Can you work these out from the drawing? Everything is in mm from the part's minimum corner. A direction names the side the tool comes from. Coordinates: 2 decimals unless noted, no trailing zeros. Order: outer loops, then holes, each group sorted by start corner. A loop starts at its lowest first (then second) coordinate and runs counter-clockwise, first axis right, second up. Notation, with made-up numbers: (31.5, 79.25) - (43.5, 79.25) arc R17 cw to (43.5, 94.25) - close; hole circle Ø1 at (1.25, 4). An arc over 180 degrees is marked (long way). Use CSV: the item, a comma, the result in double quotes. Start each with the question number.
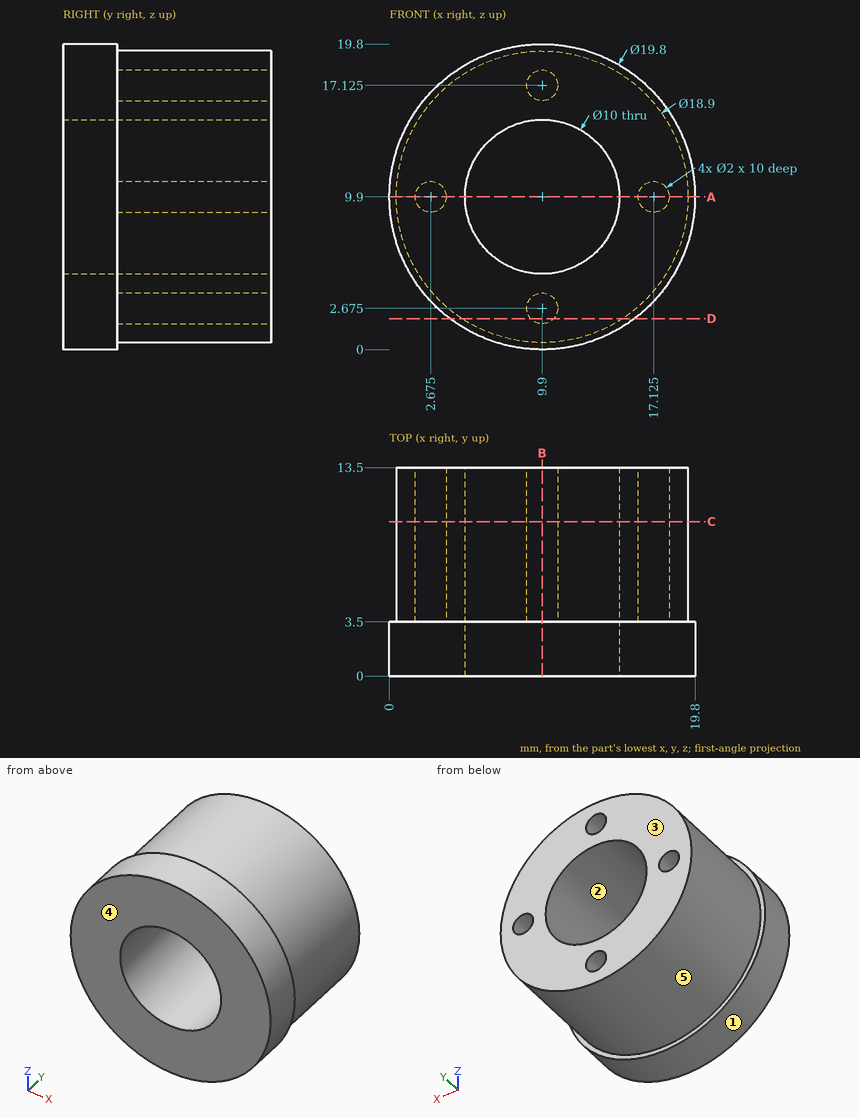
Item 1: Please list where these lines run through material, in increasing order: line 1 along Z through (x, y) = (9.9, 7) (3 decimals); line 2 along X through (y, z) = (9.5, 9). Write a range as from..to.
Item 2: Suppose I cut it at C-C on y = 10. Write out the boundary of the cut face in (x, z) (3 decimals).
Item 3: For the marked faces 4 and 5, which set-ups out of +Z, -Z, +X, -X, +Y, -Y let a thin tool reach every point of the face, with its end or its side?
Item 4: Suppose I cut it at A-A on z = 9.9. Write out the boundary of the cut face in (x, y) (3 decimals), then the cut area to 3 significant figures.
Item 5: For pin 1 Ø1.5 at (x, y) = (12, 8.5) entering from -Z; pin 2 Ø2 at (x, y) = (8, 7) entering from +Z; pin 3 Ø0.6 at (x, z) = (2.5, 10) entering from +Y, each with a flat end and sliding along its axis, tell me the tip position at first contact or that it passes through.
Item 6: We'd pull the mould along Z, two halves only. Please class the marked faces 1, 2 and 3: released by +Z, released by -Z, zero draft, split by the parting line, or undercut.
Item 7: Suppose I cut it at D-D on z = 2. Write out the boundary of the cut face in (x, y), then the cut area to 3 significant figures.
Item 8: Suppose I cut it at B-B on x = 9.9. Write out the boundary of the cut face in (y, z) (3 decimals).
Here are the results:
1,line 1,"0.45..1.675, 3.675..4.9, 14.9..16.125, 18.125..19.35"
1,line 2,"0.49..2.24, 3.11..4.98, 14.82..16.69, 17.56..19.31"
2,outline,"circle Ø18.9 at (9.9, 9.9); hole circle Ø2 at (2.675, 9.9); hole circle Ø10 at (9.9, 9.9); hole circle Ø2 at (9.9, 2.675); hole circle Ø2 at (9.9, 17.125); hole circle Ø2 at (17.125, 9.9)"
3,face 4,"+Z, -Z, +X, -X, -Y"
3,face 5,"+Y"
4,outline,"(0, 0) - (4.9, 0) - (4.9, 13.5) - (3.675, 13.5) - (3.675, 3.5) - (1.675, 3.5) - (1.675, 13.5) - (0.45, 13.5) - (0.45, 3.5) - (0, 3.5) - close; (14.9, 0) - (19.8, 0) - (19.8, 3.5) - (19.35, 3.5) - (19.35, 13.5) - (18.125, 13.5) - (18.125, 3.5) - (16.125, 3.5) - (16.125, 13.5) - (14.9, 13.5) - close"
4,area,"83.3 mm^2"
5,pin 1,"z = 0.55"
5,pin 2,"z = 19.31"
5,pin 3,"y = 3.5"
6,face 1,"split by the parting line"
6,face 2,"undercut"
6,face 3,"zero draft"
7,outline,"(3.93, 0) - (15.87, 0) - (15.87, 3.5) - (15.09, 3.5) - (15.09, 13.5) - (10.64, 13.5) - (10.64, 3.5) - (9.16, 3.5) - (9.16, 13.5) - (4.71, 13.5) - (4.71, 3.5) - (3.93, 3.5) - close"
7,area,"131 mm^2"
8,outline,"(0, 0) - (3.5, 0) - (3.5, 0.45) - (13.5, 0.45) - (13.5, 1.675) - (3.5, 1.675) - (3.5, 3.675) - (13.5, 3.675) - (13.5, 4.9) - (0, 4.9) - close; (0, 14.9) - (13.5, 14.9) - (13.5, 16.125) - (3.5, 16.125) - (3.5, 18.125) - (13.5, 18.125) - (13.5, 19.35) - (3.5, 19.35) - (3.5, 19.8) - (0, 19.8) - close"
